Design review of the part shown in the three views and the two pictorial views. Dimensions are in mm from the part's minimum x, y and z. A direction names the side the tool comes from. Coordinates: 2 decimals unless noted, no trailing zeros. Order: outer loops, then holes, each group sorted by start corner. A loop starts at its lowest first (then second) coordinate and runs counter-clockwise, first axis right, second up. Notation, with made-up numbers: (-17.75, -10) -> (-4.75, -10) arc R22 ccw to (-4.75, 15) -> close; hole circle Ø9 at (46, -1). An arc over 180 degrees is marked (long way). Answer as CSV lines item,"result". Start each with the question number.
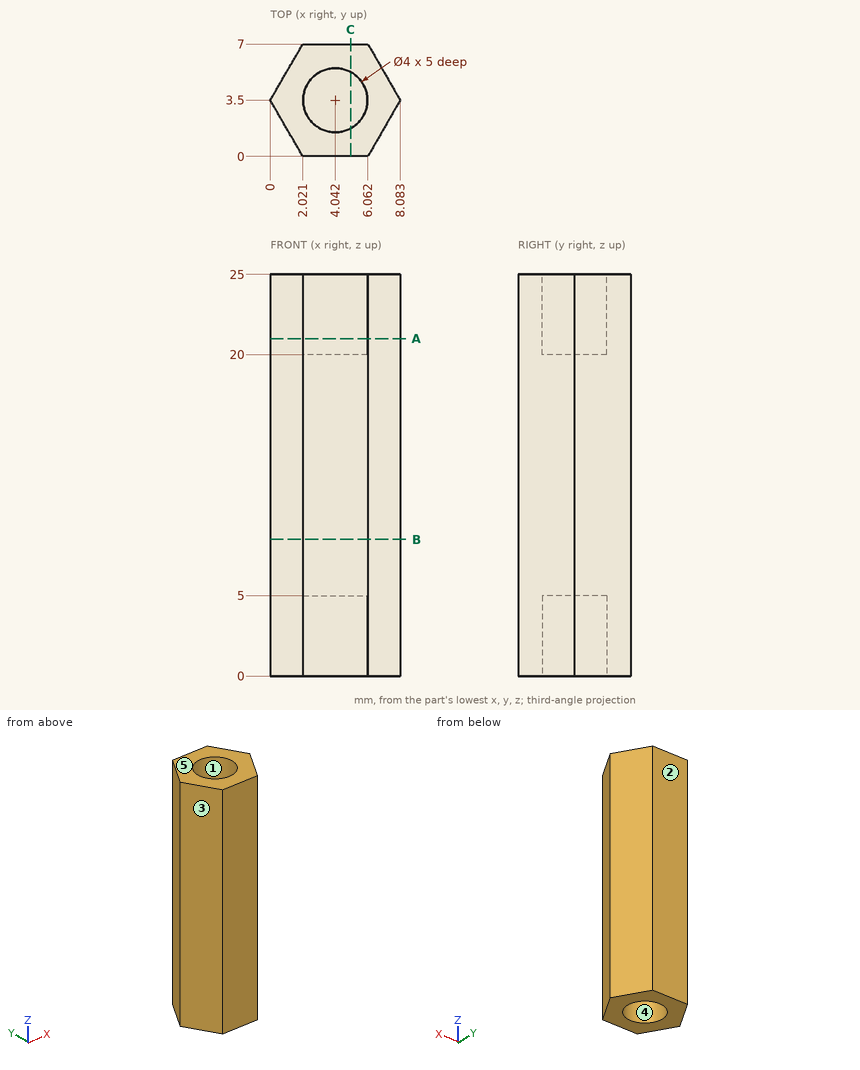
1) Wall thickness on L1, parallel to Z at x = 2.25, y = 3.25; L2, parallel to X at y = 3.25, z = 3 (1 decimal); L3, parallel to Y at x = 4.25, z = 21: over which ranges is each line inside the solid? List them lowest first. Write a range as [from, to].
2) Insertion check: pin 1 Ø2.5 at (x, y) = (4.04, 3.5) entering from -Z; pin 2 Ø1 at (y, z) = (1.5, 17) entering from +X; pin 3 Ø1.5 at (y, z) = (4, 14.5) entering from +X. Each pin has a flat end and moves straight along its axis. Give the tip position at first contact, or say it passes through.
3) Consider section B-B (z = 8.5). Give the boundary of the cut face in (x, y).
4) Consider section C-C (x = 5). Give the boundary of the cut face in (y, z) (1 decimal).
5) Tool access review of the marked faces 1 and 2: name each direction out of +Z, -Z, +X, -X, +Y, -Y from which nothing blocks a thin tool from reaching the whole face with its end or side.
6) Mouldability with a two-part tool opening along Y and no side actions: class the marked faces 3, 4 and 5 as released by +Y, released by -Y, zero draft, split by the parting line, or undercut.
7) Consider section A-A (z = 21). Give the boundary of the cut face in (x, y).
Result:
1,L1,"[5, 20]"
1,L2,"[0.1, 2.1], [6, 7.9]"
1,L3,"[0, 1.51], [5.49, 7]"
2,pin 1,"z = 5"
2,pin 2,"x = 7.22"
2,pin 3,"x = 8.08"
3,outline,"(0, 3.5) -> (2.02, 0) -> (6.06, 0) -> (8.08, 3.5) -> (6.06, 7) -> (2.02, 7) -> close"
4,outline,"(0, 0) -> (1.7, 0) -> (1.7, 5) -> (5.3, 5) -> (5.3, 0) -> (7, 0) -> (7, 25) -> (5.3, 25) -> (5.3, 20) -> (1.7, 20) -> (1.7, 25) -> (0, 25) -> close"
5,face 1,"+Z"
5,face 2,"+Z, -Z, +X, -X, +Y"
6,face 3,"released by -Y"
6,face 4,"undercut"
6,face 5,"zero draft"
7,outline,"(0, 3.5) -> (2.02, 0) -> (6.06, 0) -> (8.08, 3.5) -> (6.06, 7) -> (2.02, 7) -> close; hole circle Ø4 at (4.04, 3.5)"
